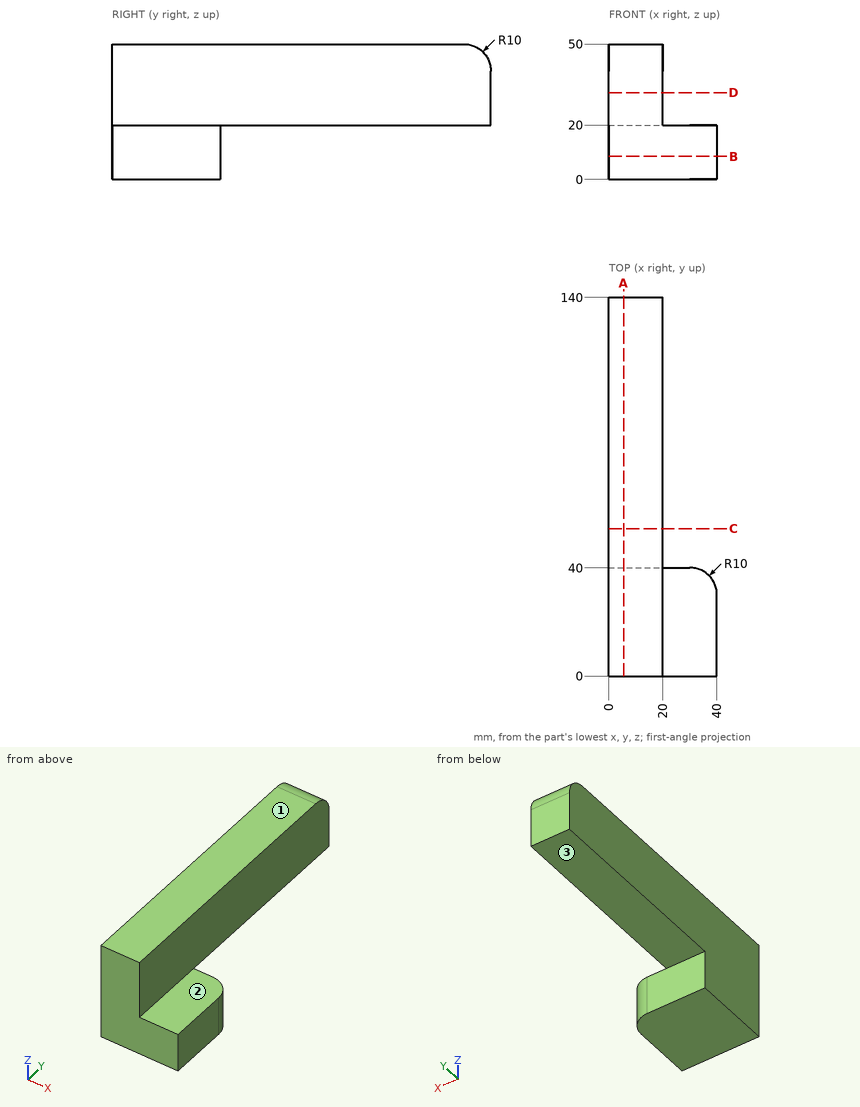
Input: dimensioned drawing with shaded views. Units: mm. Origin: part minimum x, y, z. A direction names the side the tool comes from. Round coordinates to 2 decimals unless told otherwise and drop trailing zeros. Loops run counter-clockwise (first coordinate to the right, second up) from the corner with the lowest first, then second, coordinate; pieces in that order, holes last. Notation, with made-up numbers: (56, 56.5) -> (81, 56.5) arc R15 cw to (81, 61.5) -> close; hole circle Ø9 at (0, 44). An arc over 180 degrees is marked (long way). Use one line per item in the form item = value. Start each with the question number.
1) Section D-D on z = 32. Output: boundary loops of the cut face in (x, y).
2) First-contact query: P1, Ø1.5, axis at y = 33.5, z = 33, coming from the +X side; P2, Ø8, axis at x = 21, z = 7, coming from the +Y side; P3, Ø10, axis at x = 12, y = 53, coming from the -Z side. Flat tips, straight axial feed; report the tip coordinate or a pass-through.
3) Section B-B on z = 8.5. Output: boundary loops of the cut face in (x, y).
4) Section A-A on x = 5.5. Output: boundary loops of the cut face in (y, z).
5) Section C-C on y = 54.5. Output: boundary loops of the cut face in (x, z).
6) Line query: L1, parallel to Z at x = 4, y = 42.5; L2, parallel to Y at x = 11, z = 12; L3, parallel to X at y = 66.5, z = 36.5. Output: solid intervals per line, ascending.
7) Access query for the marked faces 1, 2 and 3. Directions: +Z, -Z, +X, -X, +Y, -Y. A direction counts if a zero-diameter tool reaches every point of the face in a straight line with its end or side. Return the directions, or none.
Response:
q1.outline = (0, 0) -> (20, 0) -> (20, 140) -> (0, 140) -> close
q2.P1 = 20
q2.P2 = 40
q2.P3 = 20
q3.outline = (0, 0) -> (40, 0) -> (40, 30) arc R10 ccw to (30, 40) -> (0, 40) -> close
q4.outline = (0, 0) -> (40, 0) -> (40, 20) -> (140, 20) -> (140, 40) arc R10 ccw to (130, 50) -> (0, 50) -> close
q5.outline = (0, 20) -> (20, 20) -> (20, 50) -> (0, 50) -> close
q6.L1 = 20 to 50
q6.L2 = 0 to 40
q6.L3 = 0 to 20
q7.face_1 = +Z, +X, -X, +Y, -Y
q7.face_2 = +Z, +X, +Y, -Y
q7.face_3 = -Z, +X, -X, +Y
